Can you work these out from the model? Positions are in its coordinate system, mm. A direction names the side the tool comes from. Give positions to 0.01 mm unless a question says otherwise; leave off trailing zeros. Loops run counter-clockwise (first coordinate to the right, second up) from the corner with the lowest first, then second, coordinate; pieces in that order, holes last. Notation, with made-up numbers: (5, 55) -> (51, 55) arc R14 ccw to (51, 76) -> close; hole circle Ø5 at (29.25, 80). An arc over 180 degrees is marked (long way). Return JSON: item names as keys, results as strings. Group by question number.
Q1. Which directions (+Z, -Z, +X, -X, +Y, -Y) give clear straight access to the entire face, cutting with the end or side of a thin tool? Please do faces 5 (the flat face through (152.5, -160, 7)), 6 (the flat face through (-2, -175, 13)), 7 (the flat face through (-167.5, 160, 7)).
Q2. Thinking about a two-plate mould opening in X: for faces 1 (the flat face through (-2, 175, 13)), 2 (the flat face through (-152.5, 160, 7)), 3 (the flat face through (175, -2, 13)), 4 (the flat face through (-175, -2, 13)), which applies, pulls with the +X half, pulls with the -X half, needs draft (parallel to the pull), parting line crosses it, or undercut?
Q3. Will these pins go through, and if not, where does the flat tip stop? pin 1 (4 mm diameter, centred on x = -161, z = 4.5, fed in from +Y); pin 2 (12 mm diameter, centred on x = 156.5, y = -156, fed in from -Z); pin 3 (7 mm diameter, centred on x = -158, z = 4, fed in from -Y).
Q4. I need wall thicknesses on line 1 along Y through (x, z) = (155, 11). Which ranges of the line are inside material? Lowest first, please. Write a range as [from, to].
Q5. Suppose I cut it at A-A, the plane y = -151. Please give me the cut outline in (x, z), and give its area (3 significant figures).
```python
from build123d import *

# Parameters (mm, degrees)
SKETCH_W                = 350
SKETCH_H                = 350
PAD_DEPTH               = 27
SKETCH003_W             = 15
SKETCH003_H             = 30
POCKET_DEPTH            = 14
SKETCH003_MIRRORED_2_W  = 15
SKETCH003_MIRRORED_2_H  = 30
POCKET_MIRRORED_2_DEPTH = 14


with BuildPart() as part:
    # Sketch → Pad (new body)
    with BuildSketch(Plane.XY):
        Rectangle(SKETCH_W, SKETCH_H)
    extrude(amount=PAD_DEPTH)

    # Sketch003 (on Face5 of Pad) → Pocket (cut)
    with BuildSketch(Plane(origin=(0, 0, 0), x_dir=(1, 0, 0), z_dir=(0, 0, -1))):
        with Locations((160, -160)):
            Rectangle(SKETCH003_W, SKETCH003_H)
    pocket = extrude(amount=-POCKET_DEPTH, mode=Mode.SUBTRACT)

    # Sketch003 Mirrored 2 → Pocket Mirrored 2 (cut)
    with BuildSketch(Plane(origin=(0, 0, 0), x_dir=(-1, 0, 0), z_dir=(0, 0, 1))):
        with Locations((160, -160)):
            Rectangle(SKETCH003_MIRRORED_2_W, SKETCH003_MIRRORED_2_H)
    pocket_mirrored_2 = extrude(amount=POCKET_MIRRORED_2_DEPTH, mode=Mode.SUBTRACT)

    # Mirrored001: Pocket, Pocket Mirrored 2 across Sketch003 H_Axis
    add(pocket.mirror(Plane(origin=(0, 0, 0), x_dir=(0, 0, -1), z_dir=(0, -1, 0))), mode=Mode.SUBTRACT)
    add(pocket_mirrored_2.mirror(Plane(origin=(0, 0, 0), x_dir=(0, 0, -1), z_dir=(0, -1, 0))), mode=Mode.SUBTRACT)


solid = part.part
```
Ans:
{
 "1": {"face 5": "-Z, -Y", "face 6": "+Z, -Z, +X, -X, -Y", "face 7": "-Z, +Y"},
 "2": {"face 1": "needs draft", "face 2": "undercut", "face 3": "pulls with the +X half", "face 4": "pulls with the -X half"},
 "3": {"pin 1": "stops at y = 145", "pin 2": "stops at z = 0", "pin 3": "stops at y = -145"},
 "4": {"line 1": "y = [-145, 145]"},
 "5": {"outline": "(-175, 0) -> (-167.5, 0) -> (-167.5, 14) -> (-152.5, 14) -> (-152.5, 0) -> (152.5, 0) -> (152.5, 14) -> (167.5, 14) -> (167.5, 0) -> (175, 0) -> (175, 27) -> (-175, 27) -> close", "area": "9,030 mm^2"}
}
